Geometry: final body of the model. Coordinates: model frame, mm. Give positions to 0.01 mm unless a question says otherwise; leave off trailing zeros. Write each loop counter-clockwise with the first axis right and the second up, starting at its lowest first coordinate (ties: lowest second). Pieces come first, ordered by that corner, then holes. Notation, with made-up numbers: M 79.5,26 L 92.5,26 A14 ccw 92.5,30 Z; hole C 38.25,37.25 d6. An arc over 180 degrees is marked long. Use one line per item in the form item = value. Start each with the question number.
Item 1: Section query A-A on z = 801.5. Return loops of the section in (x, y), then the cut area to 3 significant figures.
Item 2: Contact query for flat-ended pins moving along their axis: P1, Ø4.5, axis at x = 0.5, z = 824.5, coming from the -Y side; P2, Ø1.5, axis at y = -2, z = 756.5, coming from the -X side. Output: stop coordinate, or through.
Item 3: Section query B-B on y = 1.75. Return loops of the section in (x, z).
Item 4: Material intervals for line 1 along X through (y, z) = (-0.75, 582.5); line 2 along X through (y, z) = (1.75, 64.5); line 3 along Y through (x, z) = (-2, 383), sorted ascending. Write a range as from..to.
from build123d import *

# Parameters (mm, degrees)
SKETCH1_R           = 4
BOSS_EXTRUDE1_DEPTH = 900
CUT_EXTRUDE1_START  = -3.5
SKETCH2_W           = 5.340885048
SKETCH2_H           = 17.071757563
CUT_EXTRUDE1_DEPTH  = 10


with BuildPart() as part:
    # Sketch1 → Boss-Extrude1 (new body)
    with BuildSketch(Plane.XY):
        Circle(SKETCH1_R)
    extrude(amount=BOSS_EXTRUDE1_DEPTH)

    # Sketch2 → Cut-Extrude1 (cut)
    with BuildSketch(Plane(origin=(0, 0, 0), x_dir=(1, 0, 0), z_dir=(0, 1, 0)).offset(CUT_EXTRUDE1_START)):
        with Locations((-0.042815547, -101.994282838)):
            Rectangle(SKETCH2_W, SKETCH2_H)
        with Locations((-0.042815547, -11.994282838)):
            Rectangle(SKETCH2_W, SKETCH2_H)
        with Locations((-0.042815547, -191.994282838)):
            Rectangle(SKETCH2_W, SKETCH2_H)
        with Locations((-0.042815547, -281.994282838)):
            Rectangle(SKETCH2_W, SKETCH2_H)
        with Locations((-0.042815547, -371.994282838)):
            Rectangle(SKETCH2_W, SKETCH2_H)
        with Locations((-0.042815547, -461.994282838)):
            Rectangle(SKETCH2_W, SKETCH2_H)
        with Locations((-0.042815547, -551.994282838)):
            Rectangle(SKETCH2_W, SKETCH2_H)
        with Locations((-0.042815547, -641.994282838)):
            Rectangle(SKETCH2_W, SKETCH2_H)
        with Locations((-0.042815547, -731.994282838)):
            Rectangle(SKETCH2_W, SKETCH2_H)
        with Locations((-0.042815547, -821.994282838)):
            Rectangle(SKETCH2_W, SKETCH2_H)
    extrude(amount=-CUT_EXTRUDE1_DEPTH, mode=Mode.SUBTRACT)


solid = part.part
Answer sheet:
q1.outline = C 0,0 d8
q1.area = 50.3 mm2
q2.P1 = -3.5
q2.P2 = -3.8
q3.outline = M -3.6,0 L 3.6,0 L 3.6,900 L -3.6,900 Z
q4.line_1 = -3.93..3.93
q4.line_2 = -3.6..3.6
q4.line_3 = -3.46..3.46
